CAD build for the part. Positions are in the model's coordinates, mm. Face numbers are marked on the shaded views. Coordinates: 2 decimals unless noted, no trailing zeros. Loops run counter-clockwise (first coordinate to the right, second up) from the corner with the lowest first, then second, coordinate; pieces in that order, holes last. Notation, with made-up numbers: (14.25, -37.5) -> (66.25, -37.5) arc R26 cw to (66.25, -14.5) -> close; hole circle Ø11 at (68.5, 67.25). An arc over 180 degrees is marked (long way). Write item = value, one per line. Start each with the question number.
(1) Band-saw the part on D-D (y = -52). Write the cut outline in (x, z), and give its area (3 significant figures).
(2) Drill centre lines: line 1 (Z direction, x = -0.25, y = -76); line 2 (X direction, y = -5.5, z = -61); line 3 (Y direction, x = -4, z = -138). Where is each one in solid material? Low to high. Write a range as from..to.
(3) Flat gauge pin, fed straight in: P1, Ø1.5, axis at y = 55.5, z = -64, coming from the -X side. Where does the tip first touch, or does it go through?
(4) Band-saw the part on C-C (z = 81.5). Write the cut outline in (x, y), and give its area (3 significant figures).
(5) Band-saw the part on B-B (z = 140). Write the cut outline in (x, y).
(6) Band-saw the part on A-A (y = 75). Write the cut outline in (x, z), and give its area (3 significant figures).
(7) Pull direction Z, two halves, no side cores. Call the marked faces 1 and 2: +Z half, -Z half, draft (parallel to the pull), parting line (faces both ways), or undercut.
```python
from build123d import *

# Parameters (mm, degrees)
SKICA1_W               = 350
SKICA1_H               = 200
VYSUNOUT1_DEPTH        = 10
SKICA2_R               = 15
VYSUNOUT2_DEPTH        = 5
ZAOBLIT1_R             = 1.5
LINPOLE1_COUNT         = 2
LINPOLE1_PITCH         = 280
LINPOLE1_COUNT_DIR2    = 2
LINPOLE1_PITCH_DIR2    = 150
ZAOBLIT1_OF_LINPOLE1_R = 1.5


with BuildPart() as part:
    # Skica1 → Vysunout1 (new body)
    with BuildSketch(Plane(origin=(0, 0, 0), x_dir=(0, 0, -1), z_dir=(1, 0, 0))):
        Rectangle(SKICA1_W, SKICA1_H)
    extrude(amount=VYSUNOUT1_DEPTH)

    # Skica2 → Vysunout2 (add)
    with BuildSketch(Plane.ZY):
        with Locations((-140, 75)):
            Circle(SKICA2_R)
    vysunout2 = extrude(amount=VYSUNOUT2_DEPTH)

    # Zaoblit1
    zaoblit1_edges = [part.edges().sort_by_distance(p)[0] for p in [
        (-5, 75, -155),
    ]]
    fillet(zaoblit1_edges, radius=ZAOBLIT1_R)

    # LinPole1: Vysunout2 2 × 2
    with Locations(*[(0, -j * LINPOLE1_PITCH_DIR2, i * LINPOLE1_PITCH) for i in range(LINPOLE1_COUNT) for j in range(LINPOLE1_COUNT_DIR2) if (i, j) != (0, 0)]):
        add(vysunout2)

    # Zaoblit1 of LinPole1
    zaoblit1_of_linpole1_edges = [part.edges().sort_by_distance(p)[0] for p in [
        (-5, -75, -155),
        (-5, 75, 125),
        (-5, -75, 125),
    ]]
    fillet(zaoblit1_of_linpole1_edges, radius=ZAOBLIT1_OF_LINPOLE1_R)


solid = part.part
```
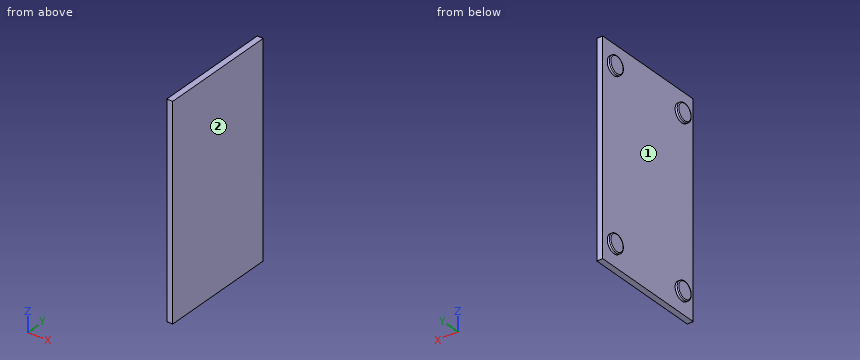
Findings below:
q1.outline = (0, -175) -> (10, -175) -> (10, 175) -> (0, 175) -> close
q1.area = 3,500 mm²
q2.line_1 = -154.97..-125.03, 125.03..154.97
q2.line_2 = 0..10
q2.line_3 = -89.78..-60.22, 60.22..89.78
q3.P1 = 0
q4.outline = (0, -100) -> (10, -100) -> (10, 100) -> (0, 100) -> close
q4.area = 2,000 mm²
q5.outline = (-5, -88.5) arc R1.5 ccw to (-3.5, -90) -> (0, -90) -> (0, -100) -> (10, -100) -> (10, 100) -> (0, 100) -> (0, 90) -> (-3.5, 90) arc R1.5 ccw to (-5, 88.5) -> (-5, 61.5) arc R1.5 ccw to (-3.5, 60) -> (0, 60) -> (0, -60) -> (-3.5, -60) arc R1.5 ccw to (-5, -61.5) -> close
q6.outline = (-5, -153.5) arc R1.5 ccw to (-3.5, -155) -> (0, -155) -> (0, -175) -> (10, -175) -> (10, 175) -> (0, 175) -> (0, 155) -> (-3.5, 155) arc R1.5 ccw to (-5, 153.5) -> (-5, 126.5) arc R1.5 ccw to (-3.5, 125) -> (0, 125) -> (0, -125) -> (-3.5, -125) arc R1.5 ccw to (-5, -126.5) -> close
q6.area = 3,800 mm²
q7.face_1 = undercut
q7.face_2 = draft
